Model file for the job. Use its own axes, mm. Face numbers are marked on the shaded views. A direction names the side the tool comes from. Give positions to 0.01 mm unless a question says otherwise; leave off trailing zeros. Order: outer loops, then holes, each group sorted by start corner. A loop starts at its lowest first (then second) coordinate and runs counter-clockwise, first axis right, second up. Notation, with made-up numbers: M -25.75,24.5 L 12.25,24.5 A15 ccw 12.25,51.5 Z; hole C 9.25,-35 d7. An arc over 180 degrees is marked long. Return JSON: item names as keys, results as strings. Group by question number.
1. Slice it at C-C on x = 23.5. List the corners of the cut face in (y, z), then the cut area to 3 significant figures.
2. Slice it at B-B on z = 22. List the corners of the cut face in (x, y).
3. Pin check, flat tips, straight feed: pin 1 (24 mm diameter, centred on x = 31, z = 24.5, fed in from +Y); pin 2 (5 mm diameter, centred on y = 7, z = 26.5, fed in from +X); pin 3 (3 mm diameter, centred on x = 43, y = 11.5, fed in from +Z). Stop position of each tip, or through.
4. 3-axis set-ups, long thin cutter, end or side, ignore diameter. For the marked faces 1, 2 and 3: which of +Z, -Z, +X, -X, +Y, -Y reach the whole face in a straight line?
5. Slice it at A-A on y = 4.5. List the corners of the cut face in (x, z), then the cut area to 3 significant figures.
6. Wall check: probe 1 along X at (y, z) = (33, 24); probe 2 along Z at (x, y) = (41.5, 15.5). Give the ranges that are in metal, low to high. Write a range as [from, to].
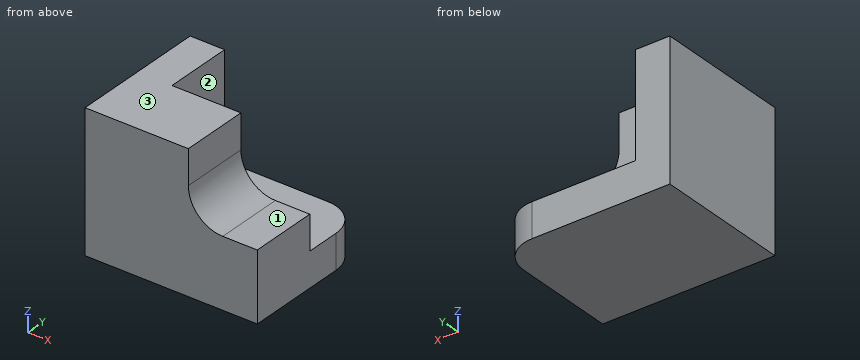
Autodesk Inventor part; units mm, degrees
ref_plane "YZ Plane" through (0, 0, 0) normal (1, 0, 0) x (0, 1, 0)
ref_plane "XZ Plane" through (0, 0, 0) normal (0, 1, 0) x (-1, 0, 0)
ref_plane "XY Plane" through (0, 0, 0) normal (0, 0, 1) x (1, 0, 0)
sketch "草圖1" plane through (0, 0, 0) normal (0, 1, 0) x (-1, 0, 0)
  line L0 (0, 0) -> (-50, 0)
  line L1 (-50, 0) -> (-50, 40)
  line L2 (-50, 40) -> (0, 40)
  line L3 (0, 40) -> (0, 0)
  dimension "d0" = 50
  dimension "d2" = 40
extrude "擠出1" add sketch "草圖1" along normal blind 40
sketch "草圖2" plane through (0, 0, 40) normal (0, 0, 1) x (1, 0, 0)
  line L0 (50, 40) -> (50, 0)
  line L1 (50, 0) -> (0, 0)
  line L2 (0, 0) -> (0, 40)
  line L3 (0, 40) -> (50, 40)
  line L4 (10, 59.2755) -> (53.3243, 59.2755)
  line L5 (53.3243, 59.2755) -> (53.3243, 20)
  line L6 (53.3243, 20) -> (10, 20)
  line L7 (10, 20) -> (10, 59.2755)
  dimension "d5" = 10
  dimension "d6" = 20
extrude "擠出2" cut sketch "草圖2" against normal blind 30 contours L3 L7 L4 L5 L6 L0 | L0 L6 L7 L3
sketch "草圖3" plane through (10, 20, 40) normal (0, 1, 0) x (1, 0, 0)
  line L0 (40, 30) -> (0, 30)
  line L1 (0, 30) -> (0, 0)
  line L2 (40, 0) -> (0, 0)
  line L3 (40, 30) -> (40, 0)
  line L4 (40, 40) -> (40, 30)
  line L5 (-10, 40) -> (40, 40)
  line L6 (-10, 0) -> (-10, 40)
  line L7 (0, 0) -> (-10, 0)
  line L8 (-10, 0) -> (40, 0)
  line L9 (40, 0) -> (20, 0)
  line L10 (20, 0) -> (20, 20)
  line L11 (20, 20) -> (40, 20)
  line L12 (40, 20) -> (40, 0)
  point P0 (20, 0)
  dimension "d9" = 20
  dimension "d10" = 20
extrude "擠出3" cut sketch "草圖3" against normal through all contours L3 L2 L10 L11
fillet "圓角1" radius 10 1 edges at (30, 10, 20)
fillet "圓角2" radius 10 1 edges at (50, 40, 5)
properties part number "36" material "鋼、碳鋼"
Result:
{
 "1": {"outline": "M 0,0 L 40,0 L 40,10 L 20,10 L 20,40 L 0,40 Z", "area": "1,000 mm2"},
 "2": {"outline": "M 0,0 L 34,0 L 34,20 L 10,20 L 10,40 L 0,40 Z"},
 "3": {"pin 1": "stops at y = 20", "pin 2": "stops at x = 32", "pin 3": "stops at z = 20"},
 "4": {"face 1": "+Z, +X, +Y, -Y", "face 2": "+Z, +X, +Y", "face 3": "+Z, +X, -X, +Y, -Y"},
 "5": {"outline": "M 0,0 L 50,0 L 50,20 L 40,20 A10 cw 30,30 L 30,40 L 0,40 Z", "area": "1,620 mm2"},
 "6": {"probe 1": "x = [0, 10]", "probe 2": "z = [0, 20]"}
}
